```python
from build123d import *

# Parameters (mm, degrees)
CROQUIS1_W              = 112
CROQUIS1_H              = 112
SALIENTE_EXTRUIR1_DEPTH = 3
CROQUIS2_W              = 50
CROQUIS2_H              = 40
SALIENTE_EXTRUIR2_DEPTH = 32
CROQUIS3_W              = 20
CROQUIS3_H              = 35
SALIENTE_EXTRUIR3_DEPTH = 18
CROQUIS4_W              = 17.5
CROQUIS4_H              = 30
CORTAR_EXTRUIR1_DEPTH   = 16
CORTAR_EXTRUIR2_DEPTH   = 46
CROQUIS6_R              = 1.5
CORTAR_EXTRUIR3_DEPTH   = 46


with BuildPart() as part:
    # Croquis1 → Saliente-Extruir1 (new body)
    with BuildSketch(Plane.XY):
        Rectangle(CROQUIS1_W, CROQUIS1_H)
    extrude(amount=SALIENTE_EXTRUIR1_DEPTH)

    # Croquis2 → Saliente-Extruir2 (add)
    with BuildSketch(Plane.XY.offset(3)):
        with Locations((24.197, -36)):
            Rectangle(CROQUIS2_W, CROQUIS2_H)
    extrude(amount=SALIENTE_EXTRUIR2_DEPTH)

    # Croquis3 → Saliente-Extruir3 (add)
    with BuildSketch(Plane.XY.offset(3)):
        with Locations((-42, 0)):
            Rectangle(CROQUIS3_W, CROQUIS3_H)
    extrude(amount=SALIENTE_EXTRUIR3_DEPTH)

    # Croquis4 → Cortar-Extruir1 (cut)
    with BuildSketch(Plane.XY.offset(21)):
        with Locations((-43.25, 0)):
            Rectangle(CROQUIS4_W, CROQUIS4_H)
    extrude(amount=-CORTAR_EXTRUIR1_DEPTH, mode=Mode.SUBTRACT)

    # Croquis5 → Cortar-Extruir2 (cut)
    with BuildSketch(Plane.XZ.offset(17.5)):
        Polygon((-52, 21), (-52, 11), (-34.000297752, 21), align=None)
    extrude(amount=-CORTAR_EXTRUIR2_DEPTH, mode=Mode.SUBTRACT)

    # Croquis6 → Cortar-Extruir3 (cut)
    with BuildSketch(Plane.XY.offset(3)):
        with Locations((-44, 46)):
            Circle(CROQUIS6_R)
        with Locations((44, 46)):
            Circle(CROQUIS6_R)
        with Locations((-6.803, -46)):
            Circle(CROQUIS6_R)
    extrude(amount=-CORTAR_EXTRUIR3_DEPTH, mode=Mode.SUBTRACT)


solid = part.part
```
CAD build for the part. Positions are in the model's coordinates, mm. A direction names the side the tool comes from. Give positions to 0.01 mm unless a question says otherwise; leave off trailing zeros. Order: outer loops, then holes, each group sorted by start corner. A loop starts at its lowest first (then second) coordinate and runs counter-clockwise, first axis right, second up.
(1) Saw through at D-D, the plane z = 15.5. Give the cut face in (x, y), then the cut area to 3 significant figures.
(2) Mould opens along Y. For faces 5 (the flat face through (24, -56, 17)), 6 (the flat face through (-41, -15, 11)), 7 (the flat face through (-56, -1, 1)) say: released by +Y, released by -Y, zero draft, split by the parting line, or undercut.
(3) Drill centre lines: L1, parallel to Y at x = 44, z = 1; L2, parallel to Y at x = -41, z = 11.5; L3, parallel to X at y = 1, z = 10. Where is each one in solid material? Low to high.
(4) Saw through at A-A, the plane x = 44. Give the cut face in (y, z).
(5) Tool access for faces 1 (the flat face through (-41, 15, 11)), 2 (the flat face through (24, -16, 19)), 3 (the flat face through (-52, 0, 4)), 4 (the flat face through (49.197, -36, 19)): list every direction of +Z, -Z, +X, -X, +Y, -Y with a clear straight run to the whole face (end or side of a thin tool).
(6) Saw through at C-C, the plane y = -46. Give the cut face in (x, z), then the cut area to 3 significant figures.
(7) Flat gauge pins, fed straight in: pin 1 (9 mm diameter, centred on y = -6, z = 8, fed in from -X); pin 2 (20 mm diameter, centred on x = -41.5, z = 8, fed in from -Y); pin 3 (14 mm diameter, centred on x = -46.5, y = -5.5, fed in from +Z); pin 4 (12.5 mm diameter, centred on x = -44, z = 11.5, fed in from -Y). Where does each tip first touch, or does it go through?
(8) Saw through at B-B, the plane y = 46. Give the cut face in (x, z).
Results found:
1. outline: (-43.9, -17.5) - (-32, -17.5) - (-32, 17.5) - (-43.9, 17.5) - (-43.9, 15) - (-34.5, 15) - (-34.5, -15) - (-43.9, -15) - close; (-0.8, -56) - (49.2, -56) - (49.2, -16) - (-0.8, -16) - close
1. area: 2,130 mm2
2. face 5: released by -Y
2. face 6: undercut
2. face 7: zero draft
3. L1: y = -56 to 44.5, 47.5 to 56
3. L2: y = -17.5 to -15, 15 to 17.5
3. L3: x = -34.5 to -32
4. outline: (-56, 0) - (44.5, 0) - (44.5, 3) - (-16, 3) - (-16, 35) - (-56, 35) - close; (47.5, 0) - (56, 0) - (56, 3) - (47.5, 3) - close
5. face 1: +Z, -X
5. face 2: +Z, +X, +Y
5. face 3: +Z, -X, +Y, -Y
5. face 4: +Z, +X, +Y, -Y
6. outline: (-56, 0) - (-8.3, 0) - (-8.3, 3) - (-56, 3) - close; (-5.3, 0) - (56, 0) - (56, 3) - (49.2, 3) - (49.2, 35) - (-0.8, 35) - (-0.8, 3) - (-5.3, 3) - close
6. area: 1,930 mm2
7. pin 1: stops at x = -52
7. pin 2: stops at y = -56
7. pin 3: stops at z = 5
7. pin 4: stops at y = -17.5
8. outline: (-56, 0) - (-45.5, 0) - (-45.5, 3) - (-56, 3) - close; (-42.5, 0) - (42.5, 0) - (42.5, 3) - (-42.5, 3) - close; (45.5, 0) - (56, 0) - (56, 3) - (45.5, 3) - close
